```python
from build123d import *

# Parameters (mm, degrees)
F0_W           = 76.2
F0_H           = 71.12
F1_DEPTH       = 73.66
F3_DEPTH       = 76.201
F4_R           = 10.16
F5_DEPTH       = 76.201
F7_DEPTH       = 71.121
F9_D           = 15.24
F9_CBORE_D     = 40.64
F9_CBORE_DEPTH = 10.16
F10_W          = 5.08
F10_H          = 10.16
F11_DEPTH      = 76.2
F12_R          = 10.16


with BuildPart() as f1:
    # F0 (on Front) → F1 (new body, symmetric)
    with BuildSketch(Plane.XZ):
        with Locations((0, 35.56)):
            Rectangle(F0_W, F0_H)
    extrude(amount=F1_DEPTH, both=True)

    # F2 (on face) → F3 (cut, through all)
    with BuildSketch(Plane.YZ.offset(38.1)):
        Polygon((38.1, 71.12), (-73.66, 71.12), (-73.66, 35.56), (2.54, 35.56), align=None)
        Polygon((38.1, 0), (73.66, 0), (73.66, 35.56), align=None)
    extrude(amount=-F3_DEPTH, mode=Mode.SUBTRACT)

    # F4 (on face) → F5 (cut, through all)
    with BuildSketch(Plane.YZ.offset(38.1)):
        with Locations((20.32, 20.32)):
            Circle(F4_R)
    extrude(amount=-F5_DEPTH, mode=Mode.SUBTRACT)

    # F6 (on face) → F7 (cut, through all)
    with BuildSketch(Plane.XY.offset(71.12)):
        with BuildLine():
            Line((22.86, 63.5), (-22.86, 63.5))
            ThreePointArc((-22.86, 63.5), (-30.48, 55.88), (-22.86, 48.26))
            Line((-22.86, 48.26), (22.86, 48.26))
            ThreePointArc((22.86, 48.26), (30.48, 55.88), (22.86, 63.5))
        make_face()
    extrude(amount=-F7_DEPTH, mode=Mode.SUBTRACT)

    # F9 (through all)
    with Locations(Plane.XY.offset(35.56)):
        with Locations((0, -35.56)):
            CounterBoreHole(F9_D / 2, F9_CBORE_D / 2, F9_CBORE_DEPTH)

    # F10 (on face) → F11 (cut)
    with BuildSketch(Plane.XZ.offset(73.66)):
        with Locations((0, 30.48)):
            Rectangle(F10_W, F10_H)
    extrude(amount=-F11_DEPTH, mode=Mode.SUBTRACT)

    # F12
    f12_edges = [f1.edges().sort_by_distance(p)[0] for p in [
        (38.1, -73.66, 17.78),
        (-38.1, -73.66, 17.78),
    ]]
    fillet(f12_edges, radius=F12_R)


solid = f1.part
```
Read the model definition and answer for the solid it produces. Units are mm, in the model's axes. A direction names the side the tool comes from. Give positions to 0.01 mm unless a question says otherwise; leave off trailing zeros. Loops run counter-clockwise (first coordinate to the right, second up) from the corner with the lowest first, then second, coordinate; pieces in that order, holes last.
Item 1: The part is cut by section A-A (x = 0). Write down the section's boundary in (y, z).
Item 2: The part is cut by section B-B (z = 54). Write down the section's boundary in (x, y).
Item 3: For faces 1 (the cylindrical face through (30.48, 55.71, 41.07)), 2 (the cylindrical face through (-20.316, -35.149, 30.551)), 3 (the flat face through (-24, -36, 35.56)), 4 (the flat face through (-2.54, -65, 30)), determine the directions among +Z, -Z, +X, -X, +Y, -Y from which every point of the face is accessible in a straight line to the end or side of a thin tool.
Item 4: The part is cut by section C-C (y = -35.56). Write down the section's boundary in (x, z), and give its area (3 significant figures).
Item 5: This flat-tipped pin is pushed along its axis until it touches: pin 1 Ø10.5 at (x, y) = (-27.5, -54.5) entering from +Z. Where does it stop, or does it pass through?
Item 6: Find the intervals of material crossed by line 1 along Y through (x, z) = (0, 20); line 2 along X through (y, z) = (-35.56, 16); line 3 along Y through (x, z) = (-7, 20), in increasing order.
Item 7: The mould has two halves that part along X. Classify faces 5 (the flat face through (38.1, 4, 27)), 6 (the flat face through (2.54, -65, 30)), 7 (the flat face through (0.53, 20.07, 53.09)): released by +X, released by -X, zero draft, split by the parting line, or undercut.
Item 8: The part is cut by section D-D (x = -16.5). Write down the section's boundary in (y, z).
Taken from the geometry:
1. outline: (-73.66, 0) - (-43.18, 0) - (-43.18, 25.4) - (-73.66, 25.4) - close; (-27.94, 0) - (38.1, 0) - (48.26, 10.16) - (48.26, 71.12) - (38.1, 71.12) - (2.54, 35.56) - (2.54, 25.4) - (-27.94, 25.4) - close; (63.5, 25.4) - (73.66, 35.56) - (73.66, 71.12) - (63.5, 71.12) - close; hole circle Ø20.32 at (20.32, 20.32)
2. outline: (-38.1, 20.98) - (38.1, 20.98) - (38.1, 73.66) - (-38.1, 73.66) - close; hole (-22.86, 48.26) - (22.86, 48.26) arc R7.62 ccw to (22.86, 63.5) - (-22.86, 63.5) arc R7.62 ccw to start
3. face 1: +Z, -Z
3. face 2: +Z
3. face 3: +Z, +X, -X, -Y
3. face 4: +Z, -Y
4. outline: (-38.1, 0) - (-7.62, 0) - (-7.62, 25.4) - (-20.32, 25.4) - (-20.32, 35.56) - (-38.1, 35.56) - close; (7.62, 0) - (38.1, 0) - (38.1, 35.56) - (20.32, 35.56) - (20.32, 25.4) - (7.62, 25.4) - close
4. area: 1,910 mm2
5. pin 1: stops at z = 35.56
6. line 1: y = -73.66 to -43.18, -27.94 to 10.17, 30.47 to 48.26
6. line 2: x = -38.1 to -7.62, 7.62 to 38.1
6. line 3: y = -73.66 to -38.57, -32.55 to 10.17, 30.47 to 48.26
7. face 5: released by +X
7. face 6: undercut
7. face 7: zero draft
8. outline: (-73.66, 0) - (38.1, 0) - (48.26, 10.16) - (48.26, 71.12) - (38.1, 71.12) - (2.54, 35.56) - (-23.7, 35.56) - (-23.7, 25.4) - (-47.42, 25.4) - (-47.42, 35.56) - (-73.66, 35.56) - close; (63.5, 25.4) - (73.66, 35.56) - (73.66, 71.12) - (63.5, 71.12) - close; hole circle Ø20.32 at (20.32, 20.32)
